The listing builds one solid part. Answer for the finished solid, in the listing's coordinates (mm). A direction names the side the tool comes from. Give positions to 0.01 mm unless a question says otherwise; leave off trailing zeros. Order: outer loops, then holes, each group sorted by start corner. A loop starts at its lowest first (then second) coordinate and runs counter-clockwise, first axis right, second up. Notation, with made-up numbers: (2.25, -14) - (52.25, -14) arc R12 ccw to (52.25, -4) - close; hole circle Ø4 at (51.25, 23). An arc over 180 degrees is marked (long way). Answer in a Markdown table with one row per item.
Autodesk Inventor part; units mm, degrees
ref_plane "YZ Plane" through (0, 0, 0) normal (1, 0, 0) x (0, 1, 0)
ref_plane "XZ Plane" through (0, 0, 0) normal (0, 1, 0) x (-1, 0, 0)
ref_plane "XY Plane" through (0, 0, 0) normal (0, 0, 1) x (1, 0, 0)
sketch "Pulley Sketch" plane through (0, 0, 0) normal (0, 0, 1) x (1, 0, 0)
  circle A0 centre (0, 0) radius 17.9
  dimension "d24" = 35.8
extrude "Extrusion3" add sketch "Pulley Sketch" along normal mid plane 10
sketch "Sketch2" plane through (0, 0, 5) normal (0, 0, 1) x (1, 0, 0)
  circle A0 centre (0, 0) radius 20
  dimension "d19" = 40
extrude "Extrusion4" add sketch "Sketch2" along normal blind 4
sketch "Sketch3" plane through (0, 0, -5) normal (0, 0, -1) x (-1, 0, 0)
  circle A0 centre (0, 0) radius 20
extrude "Extrusion5" add sketch "Sketch3" along normal blind 4
sketch "Sketch4" plane through (0, 0, -9) normal (0, 0, -1) x (-1, 0, 0)
  circle A0 centre (0, 0) radius 4
  dimension "d37" = 8
extrude "Extrusion6" cut sketch "Sketch4" against normal blind 8
sketch "Sketch5" plane through (0, 0, 9) normal (0, 0, 1) x (1, 0, 0)
  point P0 (0, 0)
  point P1 (0, 0)
hole "Hole1" at (0, 0, 9) direction (0, 0, -1) diameter 4.5 end through all
equation "\"da_pb\" = 5"
equation "\"da_fi\" = 25deg"
equation "\"da_hg\" = 1.25"
equation "\"da_bw\" = 1.8"
equation "\"da_rb\" = 0.4"
equation "\"da_rt\" = 0.6"
equation "\"da_a\" = 0.5"
equation "\"da_bf\" = 11.5"
equation "\"da_wf\" = 1"
equation "\"da_hf\" = 1.2"
properties part number "Synchronous Pulley2" material "Steel"
Item 1: Which of the six approach directions +Z, -Z, +X, -X, +Y, -Y give full straight-line access (tool end or side, diameter ignored) to faces 1 (the face through (-2, -2, -1)), 2 (the face through (14.9, -10.3, -5)), 3 (the face through (4.336, 19.524, -6.972))?
Answer block:
| item | result |
|---|---|
| face 1 | -Z |
| face 2 | none |
| face 3 | +Z, -Z |
Item 2: Each of these flat-tipped pins is pushed along its axis until it touches: P1, Ø6, axis at y = 3.5, z = 5.5, coming from the -X side; P2, Ø2, axis at x = -11.5, z = 0, coming from the +Y side; P3, Ø4, axis at y = 10.5, z = 0, coming from the +X side. Where does it stop, or does it pass through?
Answer block:
| item | result |
|---|---|
| P1 | x = -19.99 |
| P2 | y = 14.5 |
| P3 | x = 15.75 |
Item 3: Determine the mould class of faces 4 (the face through (-4.336, 19.524, 6.972)), 5 (the face through (-4.2, 0.3, -9)), 6 (the face through (0.867, -3.905, -5.056)) for opening direction Y: pulls with the +Y half, pulls with the -Y half, needs draft (parallel to the pull), parting line crosses it, or undercut.
Answer block:
| item | result |
|---|---|
| face 4 | parting line crosses it |
| face 5 | needs draft |
| face 6 | undercut |
Item 4: Find section C-C on y = -12.5. Write down the section's boundary in (x, z), then the cut area to 3 significant figures.
Answer block:
| item | result |
|---|---|
| outline | (-15.61, -9) - (15.61, -9) - (15.61, -5) - (12.81, -5) - (12.81, 5) - (15.61, 5) - (15.61, 9) - (-15.61, 9) - (-15.61, 5) - (-12.81, 5) - (-12.81, -5) - (-15.61, -5) - close |
| area | 506 mm² |
Item 5: Consider line 1 (Y direction, x = 0, z = 4.75); line 2 (Y direction, x = 0, z = -6.25); line 3 (X direction, y = 2.5, z = -2.25). Determine where each line is inside the solid, lowest interval first.
Answer block:
| item | result |
|---|---|
| line 1 | -17.9 to -2.25, 2.25 to 17.9 |
| line 2 | -20 to -4, 4 to 20 |
| line 3 | -17.72 to -3.12, 3.12 to 17.72 |
Item 6: Find section A-A on y = 0. Write down the section's boundary in (x, z).
Answer block:
| item | result |
|---|---|
| outline | (-20, -9) - (-4, -9) - (-4, -1) - (-2.25, -1) - (-2.25, 9) - (-20, 9) - (-20, 5) - (-17.9, 5) - (-17.9, -5) - (-20, -5) - close; (2.25, -1) - (4, -1) - (4, -9) - (20, -9) - (20, -5) - (17.9, -5) - (17.9, 5) - (20, 5) - (20, 9) - (2.25, 9) - close |
Item 7: Find section D-D on z = 7.75. Write down the section's boundary in (x, y), then the cut area to 3 significant figures.
Answer block:
| item | result |
|---|---|
| outline | circle Ø40 at (0, 0); hole circle Ø4.5 at (0, 0) |
| area | 1,240 mm² |
